Geometry: final body of the model. Coordinates: model frame, mm. A direction names the side the tool comes from. Give positions to 0.01 mm unless a question says otherwise; leave off trailing zeros. Write each loop counter-clockwise with the first axis right and the second up, starting at its lowest first coordinate (ties: lowest second). Pieces come first, ordered by that corner, then holes. Notation, with made-up numbers: (-35.75, 50.5) -> (-28.75, 50.5) arc R18 ccw to (-28.75, 76.5) -> close; hole circle Ø3 at (75, 40.5). An arc over 180 degrees is marked (long way). Answer in a Markdown table with one row per item. Add a question column.
Item 1: Section query C-C on y = -52. Output: boundary loops of the cut face in (x, z), plus the area to 3 significant figures.
Item 2: Section query B-B on z = 10. Output: boundary loops of the cut face in (x, y), plus the area to 3 significant figures.
Item 3: First-contact query: P1, Ø3, axis at x = 0.5, y = 29, coming from the -Z side; P2, Ø2, axis at x = -0.5, y = -6, coming from the -Z side. Flat tips, straight axial feed; report the tip coordinate or a pass-through.
Item 4: Material intervals for probe 1 along X at (y, z) = (-56.5, 7); probe 2 along Z at (x, y) = (-0.2, 49); probe 3 along Z at (x, y) = (1.3, 64.5), sorted ascending. Write a range as from..to.
Item 5: Draft query along X for faces 1 (the flat face through (-0.01, -49.41, 7.12)), 2 (the flat face through (2.5, -1, 9)), 3 (the flat face through (0, 20, 15)). Return one class per face: +X half, -X half, draft (parallel to the pull), parting line (faces both ways), or undercut.
Item 6: Access query for faces 4 (the flat face through (1.63, -55.3, 8.17)), 5 (the flat face through (0, 36, 8.676)). Directions: +Z, -Z, +X, -X, +Y, -Y. A direction counts if a zero-diameter tool reaches every point of the face in a straight line with its end or side. Return the directions, or none.
Item 7: Section query D-D on y = 18.5. Output: boundary loops of the cut face in (x, z).
```python
from build123d import *

# Parameters (mm, degrees)
F0_W        = 5
F0_H        = 150
F1_DEPTH    = 15
F2_SIZE2    = 38.4646838724
F2_SIZE     = 14
F3_T1_DEPTH = 7.1006226146
F3_T3_DEPTH = 8
F5_DEPTH    = 25
F6_T1_DEPTH = 6.5227780604
F6_T3_DEPTH = 7
F7_W        = 2
F7_H        = 30
F8_DEPTH    = 3


# Not quite as in the source:
# - a fillet or chamfer that OpenCascade refuses, or shapes differently, is made with other operations: its cross-section is extruded or revolved along the edge and cut away or added


with BuildPart() as f1:
    # F0 (on Top) → F1 (new body)
    with BuildSketch(Plane.XY):
        Rectangle(F0_W, F0_H)
    extrude(amount=F1_DEPTH)

    # F2
    f2_edges = [f1.edges().sort_by_distance(p)[0] for p in [
        (0, -75, 15),
    ]]
    f2_side = f1.faces().sort_by_distance((0, -75, 7.5))[0]
    chamfer(f2_edges, length=F2_SIZE, length2=F2_SIZE2, reference=f2_side)

    # F3: fillet of radius 0.6 on 2 edges, made by hand

    # F3_s2 → F3_t1 (cut)
    with BuildSketch(Plane.YZ.offset(-3.5503113073)):
        with BuildLine():
            ThreePointArc((-75, 0.5798754771), (-74.8914912266, 0.9240213389), (-74.605212086, 1.1436910495))
            Line((-74.605212086, 1.1436910495), (-75, 1))
            Line((-75, 1), (-75, 0.5798754771))
        make_face()
    extrude(amount=F3_T1_DEPTH, mode=Mode.SUBTRACT)

    # F3_s4 → F3_t3 (cut)
    with BuildSketch(Plane.YZ.offset(-4)):
        with BuildLine():
            ThreePointArc((-75, 0.6), (-74.8242640687, 0.1757359313), (-74.4, 0))
            Line((-74.4, 0), (-75, 0))
            Line((-75, 0), (-75, 0.6))
        make_face()
    extrude(amount=F3_T3_DEPTH, mode=Mode.SUBTRACT)

    # F4 (on face) → F5 (cut)
    with BuildSketch(Plane.YZ.offset(2.5)):
        Polygon((55, 8.6759815816), (75, 8.6759815816), (75, 15), align=None)
        with BuildLine():
            ThreePointArc((16.7323419362, 8.6759815816), (46.1873611716, 6.4950955262), (75, 0))
            Line((75, 0), (75, 8.6759815816))
            Line((75, 8.6759815816), (55, 8.6759815816))
            Line((55, 8.6759815816), (16.7323419362, 8.6759815816))
        make_face()
        with BuildLine():
            Line((-31.5353161276, 0), (75, 0))
            ThreePointArc((75, 0), (46.1873611716, 6.4950955262), (16.7323419362, 8.6759815816))
            ThreePointArc((16.7323419362, 8.6759815816), (-7.5818312879, 7.1925324796), (-31.5353161276, 2.7641913859))
            Line((-31.5353161276, 2.7641913859), (-31.5353161276, 2.76))
            Line((-31.5353161276, 2.76), (-31.5353161276, 0))
        make_face()
        Polygon((-34.0353161276, 0.69), (-31.5353161276, 0), (-31.5353161276, 2.76), (-36.5353161276, 1.38), align=None)
        Polygon((-34.0353161276, 0), (-31.5353161276, 0), (-34.0353161276, 0.69), align=None)
    extrude(amount=-F5_DEPTH, mode=Mode.SUBTRACT)

    # F6: fillet of radius 0.4 on 2 edges, made by hand

    # F6_s2 → F6_t1 (cut)
    with BuildSketch(Plane.YZ.offset(-3.2613890302)):
        with BuildLine():
            ThreePointArc((-34.0353161276, 0.3854443879), (-34.1170643339, 0.6277578125), (-34.3288951064, 0.7710277981))
            Line((-34.3288951064, 0.7710277981), (-34.0353161276, 0.69))
            Line((-34.0353161276, 0.69), (-34.0353161276, 0.3854443879))
        make_face()
    extrude(amount=F6_T1_DEPTH, mode=Mode.SUBTRACT)

    # F6_s4 → F6_t3 (cut)
    with BuildSketch(Plane.YZ.offset(-3.5)):
        with BuildLine():
            ThreePointArc((-34.4353161276, 0), (-34.1524734152, 0.1171572875), (-34.0353161276, 0.4))
            Line((-34.0353161276, 0.4), (-34.0353161276, 0))
            Line((-34.0353161276, 0), (-34.4353161276, 0))
        make_face()
    extrude(amount=F6_T3_DEPTH, mode=Mode.SUBTRACT)

    # F7 (on face) → F8 (cut)
    with BuildSketch(Plane(origin=(0, -9.0947271879, 24.9875575848), x_dir=(1, 0, 0), z_dir=(0, -0.3420201433, 0.9396926208))):
        with Locations((0, -44.2016648133)):
            Rectangle(F7_W, F7_H)
    extrude(amount=-F8_DEPTH, mode=Mode.SUBTRACT)


solid = f1.part
```
Findings below:
| question | item | result |
|---|---|---|
| 1 | outline | (-2.5, 0) -> (2.5, 0) -> (2.5, 9.37) -> (1, 9.37) -> (1, 6.18) -> (-1, 6.18) -> (-1, 9.37) -> (-2.5, 9.37) -> close |
| 1 | area | 40.5 mm^2 |
| 2 | outline | (-2.5, -50.27) -> (-1, -50.27) -> (-1, -41.5) -> (1, -41.5) -> (1, -50.27) -> (2.5, -50.27) -> (2.5, 59.19) -> (-2.5, 59.19) -> close |
| 2 | area | 530 mm^2 |
| 3 | P1 | stops at z = 8.68 |
| 3 | P2 | stops at z = 7.26 |
| 4 | probe 1 | x = -2.5..-1, 1..2.5 |
| 4 | probe 2 | z = 8.68..15 |
| 4 | probe 3 | z = 11.68..15 |
| 5 | face 1 | undercut |
| 5 | face 2 | +X half |
| 5 | face 3 | draft |
| 6 | face 4 | +Z, +X, -X, -Y |
| 6 | face 5 | -Z, +X, -X, +Y |
| 7 | outline | (-2.5, 8.68) -> (2.5, 8.68) -> (2.5, 15) -> (-2.5, 15) -> close |
